Can you work these out from the model? Positions are in its coordinate system, mm. Coordinates: 2 decimals unless noted, no trailing zeros. Order: outer loops, then holes, each group sorted by start corner. A loop starts at its lowest first (then second) coordinate and runs counter-clockwise, first axis right, second up. Notation, with made-up numbers: (49, -27) -> (79, -27) arc R27 cw to (79, -1) -> close; hole circle Ø9 at (5, 5). An arc over 180 degrees is marked (long way). Use a Markdown table: item, result. Add a question column.
1. If I drill on line 1 along X through (y, z) = (2, -195); line 2 along X through (y, z) = (8.75, -230); line 3 along Z through (x, y) = (411, 2.25), over which ranges is the centre line in solid material (lowest first)? Write a range as from..to.
2. Suppose I cut it at D-D, the plane z = -165. State how many separate pieces and enclosed holes the cut face has, then the cut area to 3 significant figures.
3. For pin 1 Ø6 at (x, y) = (518.5, 7.5) entering from -Z; pin 2 Ø3 at (y, z) = (3.5, -185.5) entering from +X; pin 3 Ø6 at (y, z) = (4.5, -254) entering from -X; pin 4 Ø8 at (x, z) = (493.5, -214) entering from +Y, each with a flat end and sliding along its axis, tell me the tip position at first contact or that it passes through.
4. Suppose I cut it at C-C, the plane y = 7. List the corners of the cut face in (x, z) for me.
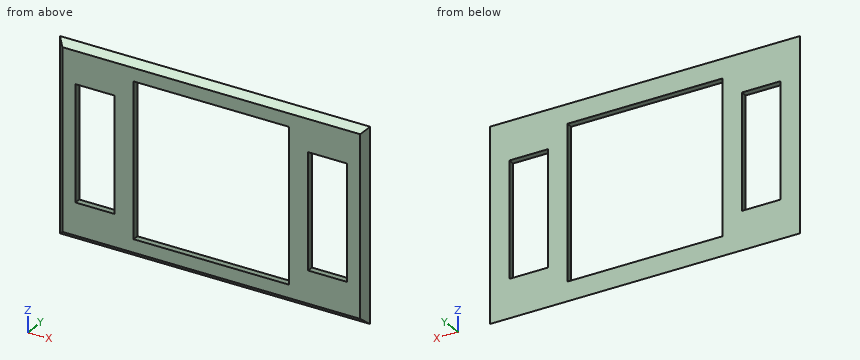
```python
from build123d import *

# Parameters (mm, degrees)
SKETCH1_W           = 75
SKETCH1_H           = 225
SKETCH1_W_2         = 300
SKETCH1_H_2         = 300
BOSS_EXTRUDE1_DEPTH = 12
CHAMFER1_SIZE       = 12


with BuildPart() as part:
    # Sketch1 → Boss-Extrude1 (new body)
    with BuildSketch(Plane(origin=(0, 0, 0), x_dir=(1, 0, 0), z_dir=(0, 1, 0))):
        Polygon((0, 375), (0, 0), (600, 0), (600, 375), (375, 375), (225, 375), align=None)
        with Locations((75, 187.5)):
            Rectangle(SKETCH1_W, SKETCH1_H, mode=Mode.SUBTRACT)
        with Locations((300, 187.5)):
            Rectangle(SKETCH1_W_2, SKETCH1_H_2, mode=Mode.SUBTRACT)
        with Locations((525, 187.5)):
            Rectangle(SKETCH1_W, SKETCH1_H, mode=Mode.SUBTRACT)
    extrude(amount=BOSS_EXTRUDE1_DEPTH)

    # Chamfer1
    chamfer1_edges = [part.edges().sort_by_distance(p)[0] for p in [
        (300, 0, -375),
        (0, 0, -187.5),
        (300, 0, 0),
        (600, 0, -187.5),
    ]]
    chamfer(chamfer1_edges, length=CHAMFER1_SIZE - 0.0001)  # a hair under: the kernel refuses the full size


solid = part.part
```
Worked out:
| question | item | result |
|---|---|---|
| 1 | line 1 | x = 10..37.5, 112.5..150, 450..487.5, 562.5..590 |
| 1 | line 2 | x = 3.25..37.5, 112.5..150, 450..487.5, 562.5..596.75 |
| 1 | line 3 | z = -365.25..-337.5, -37.5..-9.75 |
| 2 | separate pieces | 4 |
| 2 | enclosed holes | 0 |
| 2 | area | 1,660 mm² |
| 3 | pin 1 | stops at z = -373.5 |
| 3 | pin 2 | stops at x = 593 |
| 3 | pin 3 | stops at x = 4.5 |
| 3 | pin 4 | passes through |
| 4 | outline | (5, -370) -> (595, -370) -> (595, -5) -> (5, -5) -> close; hole (37.5, -300) -> (112.5, -300) -> (112.5, -75) -> (37.5, -75) -> close; hole (150, -337.5) -> (450, -337.5) -> (450, -37.5) -> (150, -37.5) -> close; hole (487.5, -300) -> (562.5, -300) -> (562.5, -75) -> (487.5, -75) -> close |
